The listing builds one solid part. Answer for the finished solid, in the listing's coordinates (mm). A direction names the side the tool comes from. Give positions to 0.01 mm unless a question says otherwise; leave off trailing zeros. Write each loop counter-clockwise with the first axis right and the second up, starting at its lowest first coordinate (ties: lowest second). Pieces come first, ordered by that corner, then holes. Notation, with made-up numbers: (-25, -20) - (19, -20) arc R15 ccw to (19, -3) - close; hole circle Ø6 at (65, 22). An arc over 180 degrees is marked (long way). One line per item, written item: value. Start each with the question number.
from build123d import *

# Parameters (mm, degrees)
F0_W     = 58.674
F0_H     = 123.698
F1_DEPTH = 7.62
F2_T     = -2.54
F4_D     = 6.35


with BuildPart() as f1:
    # F0 (on Front) → F1 (new body)
    with BuildSketch(Plane.XZ):
        with Locations((13.1707786496, -0.2674552867)):
            Rectangle(F0_W, F0_H)
    extrude(amount=F1_DEPTH)

    # F2
    f2_openings = [f1.faces().sort_by_distance(p)[0] for p in [
        (13.170779, -7.62, -0.267455),
    ]]
    offset(amount=F2_T, openings=f2_openings)

    # F4 (through all)
    with Locations(Plane(origin=(0, 0, 0), x_dir=(1, 0, 0), z_dir=(0, 1, 0))):
        with Locations((30.0433114171, -54.1525930166), (35.6767475605, -54.1525930166)):
            Hole(F4_D / 2)


solid = f1.part
Item 1: For faces 1 (the flat face through (13, -2.54, 1)), 2 (the flat face through (42.508, -4, -1)), determine the directions among +Z, -Z, +X, -X, +Y, -Y from which every point of the face is accessible in a straight line to the end or side of a thin tool.
Item 2: Find section B-B on x = 11.5. Determine the outline of the cut face in (y, z).
Item 3: Straight lines are drawn through the part: line 1 along Z through (x, y) = (13.5, -7); line 2 along X through (y, z) = (-5, 24); line 3 along Y through (x, z) = (-0.5, -36). For each, find the intervals that lie inside material, in ascending order.
Item 4: This flat-tipped pin is pushed along its axis until it touches: pin 1 Ø1 at (x, z) = (18, -15) entering from -Y. Where does it stop, or does it pass through?
Item 5: Find section A-A on z = 19. Determine the outline of the cut face in (x, y), plus the area to 3 significant figures.
Item 6: The mould has two halves that part along Z. Classify faces 3 (the flat face through (-16.166, -4, -1)), 4 (the flat face through (13, -4, -62.116)), 5 (the cylindrical face through (38.85, -1.29, 54.03)), 6 (the flat face through (13, -4, 61.582)): +Z half, -Z half, draft (parallel to the pull), parting line (faces both ways), or undercut.
Item 7: Find section C-C on y = -4.75. Determine the outline of the cut face in (x, z), plus the area to 3 significant figures.
Values:
1. face 1: -Y
1. face 2: +Z, -Z, +X, +Y, -Y
2. outline: (-7.62, -62.12) - (0, -62.12) - (0, 61.58) - (-7.62, 61.58) - (-7.62, 59.04) - (-2.54, 59.04) - (-2.54, -59.58) - (-7.62, -59.58) - close
3. line 1: -62.12 to -59.58, 59.04 to 61.58
3. line 2: -16.17 to -13.63, 39.97 to 42.51
3. line 3: -2.54 to 0
4. pin 1: y = -2.54
5. outline: (-16.17, -7.62) - (-13.63, -7.62) - (-13.63, -2.54) - (39.97, -2.54) - (39.97, -7.62) - (42.51, -7.62) - (42.51, 0) - (-16.17, 0) - close
5. area: 175 mm^2
6. face 3: draft
6. face 4: -Z half
6. face 5: undercut
6. face 6: +Z half
7. outline: (-16.17, -62.12) - (42.51, -62.12) - (42.51, 61.58) - (-16.17, 61.58) - close; hole (-13.63, -59.58) - (39.97, -59.58) - (39.97, 59.04) - (-13.63, 59.04) - close
7. area: 901 mm^2
